Can you work these out from the model? Positions are in its coordinate system, mm. Face numbers are marked on the shaded views. A direction names the side the tool comes from. Coordinates: 2 decimals unless noted, no trailing zeros. Order: outer loops, then holes, each group sorted by start corner. A loop starts at its lowest first (then second) coordinate and runs counter-clockwise, first axis right, second up. Notation, with made-up numbers: (-10, 82) -> (14, 82) arc R16 ccw to (14, 112) -> close; hole circle Ø7 at (89, 29). An arc over 180 degrees is marked (long way). Write item = value, one per line. Start each with the question number.
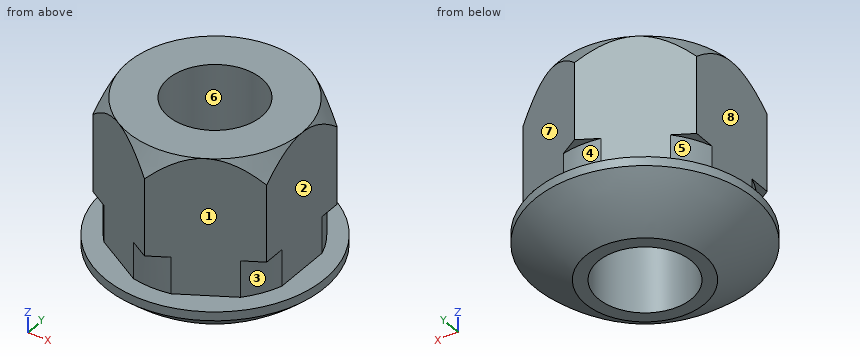
from build123d import *

# Parameters (mm, degrees)
EXTRUDE_1_DEPTH     = 15
SKETCH_2_OUTSIDE_W  = 27.534
SKETCH_2_OUTSIDE_H  = 30.474
SKETCH_2_OUTSIDE_R  = 10
CUT_EXTRUDE_1_DEPTH = 4
SKETCH_4_OUTSIDE_W  = 65.322
SKETCH_4_OUTSIDE_H  = 65.322
SKETCH_4_OUTSIDE_R  = 9.5
CUT_EXTRUDE_2_DEPTH = 27.229754265
CUT_EXTRUDE_2_DRAFT = -30
HOLE_WIZARD_M12_1_D = 10.2


with BuildPart() as part:
    # 草图1 → 凸台-拉伸1 (new body)
    with BuildSketch(Plane.XY):
        Polygon((0, 10.969655115), (-9.5, 5.484827557), (-9.5, -5.484827557), (0, -10.969655115), (9.5, -5.484827557), (9.5, 5.484827557), align=None)
    extrude(amount=-EXTRUDE_1_DEPTH)

    # 草图2 outside → 切除-拉伸1 (cut)
    with BuildSketch(Plane(origin=(0, 0, -15), x_dir=(-1, 0, 0), z_dir=(0, 0, -1))):
        Rectangle(SKETCH_2_OUTSIDE_W, SKETCH_2_OUTSIDE_H)
        Circle(SKETCH_2_OUTSIDE_R, mode=Mode.SUBTRACT)
    extrude(amount=-CUT_EXTRUDE_1_DEPTH, mode=Mode.SUBTRACT)

    # 草图3 → 旋转1 (revolve)
    with BuildSketch(Plane(origin=(0, 0, 0), x_dir=(0, 0, -1), z_dir=(1, 0, 0))):
        with BuildLine():
            Line((15, 0), (15, 12))
            Line((15, 12), (15.975879312, 12))
            ThreePointArc((15.975879312, 12), (18.176229373, 9.387763735), (20, 6.5))
            Line((20, 6.5), (20, 0))
            Line((20, 0), (15, 0))
        make_face()
    revolve(axis=Axis((0, 0, -20), (0, 0, 1)))


with BuildPart() as cut_extrude_2_tool:
    # 草图4 outside → 切除-拉伸2 (with draft: the straight prism first)
    with BuildSketch(Plane.XY):
        Rectangle(SKETCH_4_OUTSIDE_W, SKETCH_4_OUTSIDE_H)
        Circle(SKETCH_4_OUTSIDE_R, mode=Mode.SUBTRACT)
    extrude(amount=-CUT_EXTRUDE_2_DEPTH)
    # 切除-拉伸2: the draft: its side faces are tilted about the plane it starts from
    cut_extrude_2_sides = [cut_extrude_2_tool.faces().sort_by_distance(p)[0] for p in [
        (0, -32.661, -13.614877132),
        (32.661, 0, -13.614877132),
        (0, 32.661, -13.614877132),
        (-32.661, 0, -13.614877132),
        (-9.5, 0, -13.614877132),
    ]]
    draft(cut_extrude_2_sides, Plane.XY, CUT_EXTRUDE_2_DRAFT)


with BuildPart() as part_1:
    add(part.part)

    # 切除-拉伸2: cut by cut_extrude_2_tool
    add(cut_extrude_2_tool.part, mode=Mode.SUBTRACT)

    # M12 螺纹孔1 (through all)
    with Locations(Plane.XY):
        with Locations((0, 0)):
            Hole(HOLE_WIZARD_M12_1_D / 2)


solid = part_1.part
(1) Imagine slicing it at C-C (z = -1.75). Write out the boundary of the cut face in (x, y).
(2) For P1, Ø1, axis at x = -8.5, y = -5, coming from the -Z side; P2, Ø6, axis at y = 4, z = -17, coming from the -X side; P3, Ø1, axis at x = -5, z = -11, coming from the -Y side; P4, Ø9, axis at x = 0, y = 0, coming from the -Z side, each with a flat end and sliding along its axis, tell me the tip position at first contact or that it passes through.
(3) Imagine slicing it at A-A (z = -9.75). Write out the boundary of the cut face in (x, y).
(4) Imagine slicing it at B-B (z = -12.5). Write out the boundary of the cut face in (x, y).
(5) For the marked faces 1, 2, 3, 4 and 5, which set-ups out of +Z, -Z, +X, -X, +Y, -Y let a thin tool reach every point of the face, with its end or its side?
(6) If I drill on L1, parallel to X at y = -2.5, z = -8.5; L2, parallel to X at y = 0.75, z = -18; L3, parallel to Y at x = -3.5, z = -14.75, over which ranges is the centre line in solid material (lowest first)? Write a range as from..to.
(7) Thinking about a two-plate mould opening in X: for the marked faces 6, 7 and 8, which applies, +X half, -X half, draft (parallel to the pull), parting line (faces both ways), or undercut?
Result set:
q1.outline = (-9.5, -4.5) arc R10.51 ccw to (-8.64, -5.98) -> (-0.86, -10.48) arc R10.51 ccw to (0.86, -10.48) -> (8.64, -5.98) arc R10.51 ccw to (9.5, -4.5) -> (9.5, 4.5) arc R10.51 ccw to (8.64, 5.98) -> (0.86, 10.48) arc R10.51 ccw to (-0.86, 10.48) -> (-8.64, 5.98) arc R10.51 ccw to (-9.5, 4.5) -> close; hole circle Ø10.2 at (0, 0)
q2.P1 = -18.2
q2.P2 = -11.94
q2.P3 = -8.37
q2.P4 = through
q3.outline = (-9.5, -5.48) -> (0, -10.97) -> (9.5, -5.48) -> (9.5, 5.48) -> (0, 10.97) -> (-9.5, 5.48) -> close; hole circle Ø10.2 at (0, 0)
q4.outline = (-9.5, -3.12) arc R10 ccw to (-7.45, -6.67) -> (-2.05, -9.79) arc R10 ccw to (2.05, -9.79) -> (7.45, -6.67) arc R10 ccw to (9.5, -3.12) -> (9.5, 3.12) arc R10 ccw to (7.45, 6.67) -> (2.05, 9.79) arc R10 ccw to (-2.05, 9.79) -> (-7.45, 6.67) arc R10 ccw to (-9.5, 3.12) -> close; hole circle Ø10.2 at (0, 0)
q5.face_1 = +Z, +X, -Y
q5.face_2 = +Z, +X, +Y, -Y
q5.face_3 = +X, -Y
q5.face_4 = +Y
q5.face_5 = -X, +Y
q6.L1 = -9.5..-4.45, 4.45..9.5
q6.L2 = -9.6..-5.04, 5.04..9.6
q6.L3 = -8.95..-3.71, 3.71..8.95
q7.face_6 = undercut
q7.face_7 = +X half
q7.face_8 = -X half
